Model file for the job. Use its own axes, mm. Round coordinates to 2 decimals unless told otherwise and drop trailing zeros. Order: outer loops, then holes, each group sorted by start corner. A loop starts at its lowest first (then second) coordinate and runs counter-clockwise, first axis right, second up. Notation, with made-up numbers: (37, 27.25) -> (53, 27.25) arc R21 cw to (53, 59.25) -> close; hole circle Ø6 at (-37.75, -23). An arc over 180 degrees is marked (long way). Put each result on its own line as item: value. Start each with the question number.
Q1. Probe L1, parallel to Z at x = 0, y = -21.5 (3 decimals); L2, parallel to Z at x = -12, y = -23; L3, parallel to X at y = -21, z = 641. List the from-to ranges inside material, lowest first.
Q2. Cut at A-A, the plane z = 506. List the corners of the cut face in (x, y).
Q3. Cut at B-B, the plane y = 5. List the corners of the cut face in (x, z).
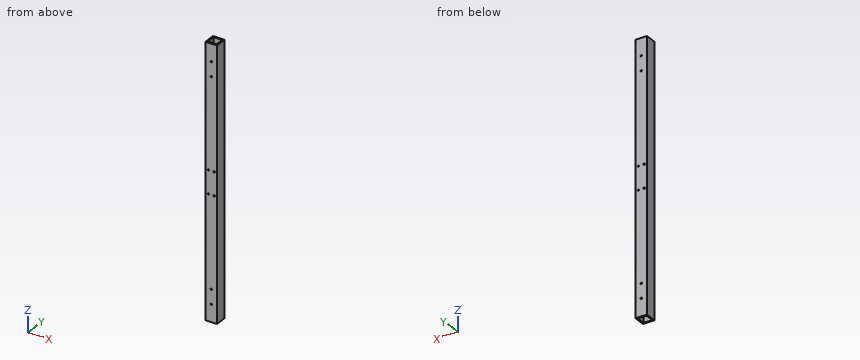
from build123d import *

# Parameters (mm, degrees)
SKETCH1_W                   = 50.8
SKETCH1_H                   = 50.8
BOSS_EXTRUDE1_DEPTH         = 1181.1
SKETCH8_W                   = 38.1
SKETCH8_H                   = 38.1
CUT_EXTRUDE1_DEPTH          = 1182.1
F_1_4_0_25_DIAMETER_HOLE1_D = 6.35
E_0_25_DIAMETER_HOLE2_D     = 6.35


with BuildPart() as part:
    # Sketch1 → Boss-Extrude1 (new body)
    with BuildSketch(Plane.XY):
        Rectangle(SKETCH1_W, SKETCH1_H)
    extrude(amount=BOSS_EXTRUDE1_DEPTH)

    # Sketch8 → Cut-Extrude1 (cut, through all)
    with BuildSketch(Plane.XY.offset(1181.1)):
        Rectangle(SKETCH8_W, SKETCH8_H)
    extrude(amount=-CUT_EXTRUDE1_DEPTH, mode=Mode.SUBTRACT)

    # 1/4 (0.25) Diameter Hole1 (through all)
    with Locations(Plane(origin=(0, 25.4, 0), x_dir=(1, 0, 0), z_dir=(0, 1, 0))):
        with Locations((-12.7, -641.35), (12.7, -641.35), (12.7, -539.75), (-12.7, -539.75)):
            Hole(F_1_4_0_25_DIAMETER_HOLE1_D / 2)

    # E (0.25) Diameter Hole2 (through all)
    with Locations(Plane(origin=(0, 25.4, 0), x_dir=(1, 0, 0), z_dir=(0, 1, 0))):
        with Locations((0, -1104.9), (0, -1041.4), (0, -139.7), (0, -76.2)):
            Hole(E_0_25_DIAMETER_HOLE2_D / 2)


solid = part.part
Ans:
1. L1: z = 0 to 73.025, 79.375 to 136.525, 142.875 to 1038.225, 1044.575 to 1101.725, 1108.075 to 1181.1
1. L2: z = 0 to 536.65, 542.85 to 638.25, 644.45 to 1181.1
1. L3: x = -25.4 to -15.86, -9.54 to 9.54, 15.86 to 25.4
2. outline: (-25.4, -25.4) -> (25.4, -25.4) -> (25.4, 25.4) -> (-25.4, 25.4) -> close; hole (-19.05, -19.05) -> (19.05, -19.05) -> (19.05, 19.05) -> (-19.05, 19.05) -> close
3. outline: (-25.4, 0) -> (-19.05, 0) -> (-19.05, 1181.1) -> (-25.4, 1181.1) -> close; (19.05, 0) -> (25.4, 0) -> (25.4, 1181.1) -> (19.05, 1181.1) -> close
